from build123d import *

# Parameters (mm, degrees)
F0_R     = 20
F0_R_2   = 15
F1_DEPTH = 2.5


# Not quite as in the source:
# - a fillet or chamfer that OpenCascade refuses, or shapes differently, is made with other operations: its cross-section is extruded or revolved along the edge and cut away or added


with BuildPart() as f1:
    # F0 (on Front) → F1 (new body)
    with BuildSketch(Plane.XZ):
        Circle(F0_R)
        Circle(F0_R_2, mode=Mode.SUBTRACT)
    extrude(amount=F1_DEPTH)

    # F2: fillet of radius 5 on 1 edges, made by hand

    # F2_s1 → F2_t2 (revolve, cut)
    with BuildSketch(Plane.XY):
        with BuildLine():
            ThreePointArc((20, 0), (18.1698729811, -1.8301270189), (15.6698729811, -2.5))
            Line((15.6698729811, -2.5), (20, -2.5))
            Line((20, -2.5), (20, 0))
        make_face()
    revolve(axis=Axis((0, -2.5, 0), (0, -1, 0)), mode=Mode.SUBTRACT)

    # F3: F1 across plane


with BuildPart() as f1_1:
    add(f1.part)
    add(f1.part.mirror(Plane.XZ))


solid = f1_1.part
Geometry: final body of the model. Coordinates: model frame, mm. Give positions to 0.01 mm unless a question says otherwise; leave off trailing zeros. Write each loop counter-clockwise with the first axis right and the second up, starting at its lowest first coordinate (ties: lowest second). Pieces come first, ordered by that corner, then holes. Notation, with made-up numbers: (-9, -29.5) -> (24, -29.5) arc R34 cw to (24, 2.5) -> close; hole circle Ø10 at (49, 2.5). An arc over 180 degrees is marked (long way). Answer in a Markdown table with one row per item.
(1) Section query C-C on y = -1.1. Return loops of the section in (x, z), then the cut area to 3 significant figures.
Answers below:
| item | result |
|---|---|
| outline | circle Ø38.28 at (0, 0); hole circle Ø30 at (0, 0) |
| area | 444 mm^2 |
(2) Section query A-A on x = 0. Return loops of the section in (y, z), then the cut area to 3 significant figures.
Answers below:
| item | result |
|---|---|
| outline | (-2.5, -15.67) arc R5 ccw to (0, -20) arc R5 ccw to (2.5, -15.67) -> (2.5, -15) -> (-2.5, -15) -> close; (-2.5, 15) -> (2.5, 15) -> (2.5, 15.67) arc R5 ccw to (0, 20) arc R5 ccw to (-2.5, 15.67) -> close |
| area | 37.4 mm^2 |
(3) Section query B-B on z = 0. Return loops of the section in (x, y).
Answers below:
| item | result |
|---|---|
| outline | (-20, 0) arc R5 ccw to (-15.67, -2.5) -> (-15, -2.5) -> (-15, 2.5) -> (-15.67, 2.5) arc R5 ccw to start; (15, -2.5) -> (15.67, -2.5) arc R5 ccw to (20, 0) arc R5 ccw to (15.67, 2.5) -> (15, 2.5) -> close |
(4) Ray query, line 1 along X through (y, z) = (0.9, -6); line 2 along X through (y, z) = (-1.3, -10.5); line 3 along Z through (x, y) = (0, -0.75). Return the intervals inside material, ascending. Write a range as [from, to].
Answers below:
| item | result |
|---|---|
| line 1 | [-18.38, -13.75], [13.75, 18.38] |
| line 2 | [-15.74, -10.71], [10.71, 15.74] |
| line 3 | [-19.47, -15], [15, 19.47] |
(5) Pin query (flat end, axial travel): pin 1 (1.5 mm diameter, centred on y = -1, z = 4, fed in from +X). Return the tip coordinate at first contact, or that it passes through.
Answers below:
| item | result |
|---|---|
| pin 1 | x = 19.46 |
